```python
from build123d import *

# Parameters (mm, degrees)
SKETCH_223_R             = 11.5
SKETCH_223_R_2           = 8.5
EXTRUDE_6_DEPTH          = 11.5
SKETCH_7_R               = 11.5
EXTRUDE_7_DEPTH          = 15
CUT_EXTRUDE_1_REACH      = 36.373
CUT_EXTRUDE_1_END_RADIUS = 11.5
SKETCH_4_W               = 5
SKETCH_4_H               = 10
SKETCH_1_W               = 35
SKETCH_1_H               = 26.5
SKETCH_1_W_2             = 27
SKETCH_1_H_2             = 63
SKETCH_1_R               = 2.5
EXTRUDE_8_DEPTH          = 1.5
SKETCH_1_5_W             = 27
SKETCH_1_5_H             = 63
SKETCH_1_5_W_2           = 35
SKETCH_1_5_H_2           = 26.5
EXTRUDE_9_DEPTH          = 25
SKETCH_1_6_R             = 2.5
SKETCH_1_6_R_2           = 1.25
EXTRUDE_10_DEPTH         = 8
EXTRUDE_11_DEPTH         = 15
SKETCH_1_9_R             = 2
SKETCH_1_9_R_2           = 1.25
EXTRUDE_22_DEPTH         = 15
CUT_EXTRUDE_2_REACH      = 81.456
SKETCH_5_W               = 28
SKETCH_5_H               = 13
CUT_EXTRUDE_3_REACH      = 81.687
SKETCH_6_W               = 25
SKETCH_6_H               = 13
CUT_EXTRUDE_4_REACH      = 98.628


with BuildPart() as part:
    # Sketch 223 → Extrude 6 (new body)
    with BuildSketch(Plane(origin=(0, 0, 0), x_dir=(1, 0, 0), z_dir=(0, 1, 0))):
        with Locations(Location((14, 14, 0), (0, 0, 270))):
            Circle(SKETCH_223_R)
        with Locations(Location((14, 14, 0), (0, 0, 270))):
            Circle(SKETCH_223_R_2, mode=Mode.SUBTRACT)
    extrude(amount=EXTRUDE_6_DEPTH)

    # Sketch 7 → Extrude 7 (add)
    with BuildSketch(Plane(origin=(0, 0, 0), x_dir=(1, 0, 0), z_dir=(0, 1, 0))):
        with Locations(Location((14, 14, 0), (0, 0, 270))):
            Circle(SKETCH_7_R)
        with BuildLine():
            ThreePointArc((21.892872757, 19.724077187), (23.274103983, 17.008902675), (23.75, 14))
            ThreePointArc((23.75, 14), (21.390430568, 7.640437435), (15.453787483, 4.358993727))
            ThreePointArc((15.453787483, 4.358993727), (13.954467258, 3.002614207), (12.466429945, 4.371362356))
            ThreePointArc((12.466429945, 4.371362356), (4.976803671, 10.306163512), (6.1547961, 19.789237926))
            ThreePointArc((6.1547961, 19.789237926), (6.255870441, 21.80852258), (8.275922813, 21.892872757))
            ThreePointArc((8.275922813, 21.892872757), (14.040367815, 23.749916432), (19.789237926, 21.8452039))
            ThreePointArc((19.789237926, 21.8452039), (21.80852258, 21.744129559), (21.892872757, 19.724077187))
        make_face(mode=Mode.SUBTRACT)
    extrude(amount=EXTRUDE_7_DEPTH)

    # Cut-Extrude 1: up to this cylinder (the profile starts inside it)
    cut_extrude_1_end = Plane(origin=(14, 5, -14), z_dir=(0, -1, 0)) * Cylinder(CUT_EXTRUDE_1_END_RADIUS, 96.746, mode=Mode.PRIVATE)
    # Sketch 4 → Cut-Extrude 1 (cut, up to the surface)
    with BuildSketch(Plane.XY.offset(-20), mode=Mode.PRIVATE) as cut_extrude_1_sk1:
        with Locations((14.03258037, 5)):
            Rectangle(SKETCH_4_W, SKETCH_4_H)
    cut_extrude_1_tool1 = extrude(cut_extrude_1_sk1.sketch, amount=-CUT_EXTRUDE_1_REACH, mode=Mode.PRIVATE) & cut_extrude_1_end
    add(cut_extrude_1_tool1.solids().sort_by_distance((14.03258, 5, -20))[0], mode=Mode.SUBTRACT)

    # Sketch 1 → Extrude 8 (add)
    # profile 1 of 3: a face of its own
    with BuildSketch(Plane(origin=(0, 0, 0), x_dir=(1, 0, 0), z_dir=(0, 1, 0))):
        with Locations((19, 51.25)):
            Rectangle(SKETCH_1_W, SKETCH_1_H)
    # profile 2 of 3: a face of its own
    with BuildSketch(Plane(origin=(0, 0, 0), x_dir=(1, 0, 0), z_dir=(0, 1, 0))):
        with BuildLine():
            ThreePointArc((3.5, 37), (4.914213562, 33.585786438), (1.5, 35))
            Line((1.5, 35), (1.5, 3.5))
            ThreePointArc((1.5, 3.5), (4.914213562, 4.914213562), (3.5, 1.5))
            Line((3.5, 1.5), (34.5, 1.5))
            ThreePointArc((34.5, 1.5), (33.085786438, 4.914213562), (36.5, 3.5))
            Line((36.5, 3.5), (36.5, 35))
            ThreePointArc((36.5, 35), (33.085786438, 33.585786438), (34.5, 37))
            Line((34.5, 37), (3.5, 37))
        make_face()
    # profile 3 of 3: a face of its own
    with BuildSketch(Plane(origin=(0, 0, 0), x_dir=(1, 0, 0), z_dir=(0, 1, 0))):
        with Locations((51, 33)):
            Rectangle(SKETCH_1_W_2, SKETCH_1_H_2)
        with Locations(Location((40.9, 15.6, 0), (0, 0, 270))):
            Circle(SKETCH_1_R, mode=Mode.SUBTRACT)
        with Locations(Location((61.1, 15.6, 0), (0, 0, 270))):
            Circle(SKETCH_1_R, mode=Mode.SUBTRACT)
        with Locations(Location((40.9, 61.1, 0), (0, 0, 270))):
            Circle(SKETCH_1_R, mode=Mode.SUBTRACT)
        with Locations(Location((61.1, 61.1, 0), (0, 0, 270))):
            Circle(SKETCH_1_R, mode=Mode.SUBTRACT)
    extrude(amount=EXTRUDE_8_DEPTH)


with BuildPart() as extrude_8_piece_1:
    # of the separate pieces the step leaves, piece 1, a body of its own (extrude_8_pieces)
    add(part.part.solids().sort_by_distance((14, 15, -2.5))[0])



with BuildPart() as extrude_8_piece_2:
    # of the separate pieces the step leaves, piece 2, a body of its own (extrude_8_pieces)
    add(part.part.solids().sort_by_distance((37.5, 0, -1.5))[0])



with BuildPart() as extrude_8_piece_3:
    # of the separate pieces the step leaves, piece 3, a body of its own (extrude_8_pieces)
    add(part.part.solids().sort_by_distance((1.5, 0, -64.5))[0])


with BuildPart() as extrude_8_piece_2_1:
    add(extrude_8_piece_2.part)

    add(extrude_8_piece_3.part)  # Extrude 9 merges Extrude 8 piece 3
    # Sketch 1_5 → Extrude 9 (add)
    with BuildSketch(Plane(origin=(0, 0, 0), x_dir=(1, 0, 0), z_dir=(0, 1, 0))):
        Polygon((0, 37), (36.5, 37), (36.5, 0), (66, 0), (66, 66), (0, 66), align=None)
        with Locations((51, 33)):
            Rectangle(SKETCH_1_5_W, SKETCH_1_5_H, mode=Mode.SUBTRACT)
        with Locations((19, 51.25)):
            Rectangle(SKETCH_1_5_W_2, SKETCH_1_5_H_2, mode=Mode.SUBTRACT)
    extrude(amount=EXTRUDE_9_DEPTH)

    # Sketch 1_6 → Extrude 10 (add)
    # profile 1 of 4: a face of its own
    with BuildSketch(Plane(origin=(0, 0, 0), x_dir=(1, 0, 0), z_dir=(0, 1, 0))):
        with Locations(Location((61.1, 61.1, 0), (0, 0, 270))):
            Circle(SKETCH_1_6_R)
        with Locations(Location((61.1, 61.1, 0), (0, 0, 270))):
            Circle(SKETCH_1_6_R_2, mode=Mode.SUBTRACT)
    # profile 2 of 4: a face of its own
    with BuildSketch(Plane(origin=(0, 0, 0), x_dir=(1, 0, 0), z_dir=(0, 1, 0))):
        with Locations(Location((40.9, 61.1, 0), (0, 0, 270))):
            Circle(SKETCH_1_6_R)
        with Locations(Location((40.9, 61.1, 0), (0, 0, 270))):
            Circle(SKETCH_1_6_R_2, mode=Mode.SUBTRACT)
    # profile 3 of 4: a face of its own
    with BuildSketch(Plane(origin=(0, 0, 0), x_dir=(1, 0, 0), z_dir=(0, 1, 0))):
        with Locations(Location((40.9, 15.6, 0), (0, 0, 270))):
            Circle(SKETCH_1_6_R)
        with Locations(Location((40.9, 15.6, 0), (0, 0, 270))):
            Circle(SKETCH_1_6_R_2, mode=Mode.SUBTRACT)
    # profile 4 of 4: a face of its own
    with BuildSketch(Plane(origin=(0, 0, 0), x_dir=(1, 0, 0), z_dir=(0, 1, 0))):
        with Locations(Location((61.1, 15.6, 0), (0, 0, 270))):
            Circle(SKETCH_1_6_R)
        with Locations(Location((61.1, 15.6, 0), (0, 0, 270))):
            Circle(SKETCH_1_6_R_2, mode=Mode.SUBTRACT)
    extrude(amount=EXTRUDE_10_DEPTH)


with BuildPart() as extrude_8_piece_1_1:
    add(extrude_8_piece_1.part)

    add(extrude_8_piece_2_1.part)  # Extrude 11 merges Extrude 8 piece 2
    # Sketch 1_7 → Extrude 11 (add)
    with BuildSketch(Plane(origin=(0, 0, 0), x_dir=(1, 0, 0), z_dir=(0, 1, 0))):
        Polygon((1.5, 35), (1.5, 37), (0, 37), (0, 0), (36.5, 0), (36.5, 1.5), (34.5, 1.5), (3.5, 1.5), (1.5, 1.5), (1.5, 3.5), align=None)
    extrude(amount=EXTRUDE_11_DEPTH)

    # Sketch 1_9 → Extrude 22 (add)
    # profile 1 of 8: a face of its own
    with BuildSketch(Plane(origin=(0, 0, 0), x_dir=(1, 0, 0), z_dir=(0, 1, 0))):
        with Locations((3.5, 3.5)):
            Circle(SKETCH_1_9_R)
        with Locations(Location((3.5, 3.5, 0), (0, 0, 270))):
            Circle(SKETCH_1_9_R_2, mode=Mode.SUBTRACT)
    # profile 2 of 8: a face of its own
    with BuildSketch(Plane(origin=(0, 0, 0), x_dir=(1, 0, 0), z_dir=(0, 1, 0))):
        with BuildLine():
            ThreePointArc((3.5, 1.5), (2.085786438, 2.085786438), (1.5, 3.5))
            Line((1.5, 3.5), (1.5, 1.5))
            Line((1.5, 1.5), (3.5, 1.5))
        make_face()
    # profile 3 of 8: a face of its own
    with BuildSketch(Plane(origin=(0, 0, 0), x_dir=(1, 0, 0), z_dir=(0, 1, 0))):
        with Locations((34.5, 3.5)):
            Circle(SKETCH_1_9_R)
        with Locations(Location((34.5, 3.5, 0), (0, 0, 270))):
            Circle(SKETCH_1_9_R_2, mode=Mode.SUBTRACT)
    # profile 4 of 8: a face of its own
    with BuildSketch(Plane(origin=(0, 0, 0), x_dir=(1, 0, 0), z_dir=(0, 1, 0))):
        with BuildLine():
            ThreePointArc((36.5, 3.5), (35.914213562, 2.085786438), (34.5, 1.5))
            Line((34.5, 1.5), (36.5, 1.5))
            Line((36.5, 1.5), (36.5, 3.5))
        make_face()
    # profile 5 of 8: a face of its own
    with BuildSketch(Plane(origin=(0, 0, 0), x_dir=(1, 0, 0), z_dir=(0, 1, 0))):
        with Locations((34.5, 35)):
            Circle(SKETCH_1_9_R)
        with Locations(Location((34.5, 35, 0), (0, 0, 270))):
            Circle(SKETCH_1_9_R_2, mode=Mode.SUBTRACT)
    # profile 6 of 8: a face of its own
    with BuildSketch(Plane(origin=(0, 0, 0), x_dir=(1, 0, 0), z_dir=(0, 1, 0))):
        with BuildLine():
            Line((36.5, 37), (34.5, 37))
            ThreePointArc((34.5, 37), (35.914213562, 36.414213562), (36.5, 35))
            Line((36.5, 35), (36.5, 37))
        make_face()
    # profile 7 of 8: a face of its own
    with BuildSketch(Plane(origin=(0, 0, 0), x_dir=(1, 0, 0), z_dir=(0, 1, 0))):
        with Locations((3.5, 35)):
            Circle(SKETCH_1_9_R)
        with Locations(Location((3.5, 35, 0), (0, 0, 270))):
            Circle(SKETCH_1_9_R_2, mode=Mode.SUBTRACT)
    # profile 8 of 8: a face of its own
    with BuildSketch(Plane(origin=(0, 0, 0), x_dir=(1, 0, 0), z_dir=(0, 1, 0))):
        with BuildLine():
            Line((3.5, 37), (1.5, 37))
            Line((1.5, 37), (1.5, 35))
            ThreePointArc((1.5, 35), (2.085786438, 36.414213562), (3.5, 37))
        make_face()
    extrude(amount=EXTRUDE_22_DEPTH)

    # Sketch 5 → Cut-Extrude 2 (cut, up to next)
    with BuildSketch(Plane.ZY.offset(-36.5), mode=Mode.PRIVATE) as cut_extrude_2_sk1:
        with Locations((-18.5, 8)):
            Rectangle(SKETCH_5_W, SKETCH_5_H)
    cut_extrude_2_tool1 = extrude(cut_extrude_2_sk1.sketch, amount=-CUT_EXTRUDE_2_REACH, mode=Mode.PRIVATE) & extrude_8_piece_1_1.part
    add(cut_extrude_2_tool1.solids().sort_by_distance((36.5, 8, -18.5))[0], mode=Mode.SUBTRACT)

    # Sketch 6 → Cut-Extrude 3 (cut, up to next)
    with BuildSketch(Plane.XY.offset(-37), mode=Mode.PRIVATE) as cut_extrude_3_sk1:
        with Locations((20, 8)):
            Rectangle(SKETCH_6_W, SKETCH_6_H)
    cut_extrude_3_tool1 = extrude(cut_extrude_3_sk1.sketch, amount=-CUT_EXTRUDE_3_REACH, mode=Mode.PRIVATE) & extrude_8_piece_1_1.part
    add(cut_extrude_3_tool1.solids().sort_by_distance((20, 8, -37))[0], mode=Mode.SUBTRACT)

    # Sketch 7 2 → Cut-Extrude 4 (cut, up to next)
    with BuildSketch(Plane.ZY, mode=Mode.PRIVATE) as cut_extrude_4_sk1:
        with BuildLine():
            Line((-57.5, 10.5), (-45.5, 10.5))
            ThreePointArc((-45.5, 10.5), (-43, 8), (-45.5, 5.5))
            Line((-45.5, 5.5), (-57.5, 5.5))
            ThreePointArc((-57.5, 5.5), (-60, 8), (-57.5, 10.5))
        make_face()
    cut_extrude_4_tool1 = extrude(cut_extrude_4_sk1.sketch, amount=-CUT_EXTRUDE_4_REACH, mode=Mode.PRIVATE) & extrude_8_piece_1_1.part
    add(cut_extrude_4_tool1.solids().sort_by_distance((0, 8, -51.5))[0], mode=Mode.SUBTRACT)


solid = extrude_8_piece_1_1.part
```
Read the model definition and answer for the solid it produces. Units are mm, in the model's axes. A direction names the side the tool comes from. Coordinates: 2 decimals unless noted, no trailing zeros. Loops run counter-clockwise (first coordinate to the right, second up) from the corner with the lowest first, then second, coordinate; pieces in that order, holes last.
(1) A tool of negligible diameter and unlimited length cuts with its end or side. For faces 3 (the face through (11.533, 6, -24)), 4 (the face through (17.45, 8.16, -3.03)), 5 (the face through (1, 10.5, -52)), from which of +Z, -Z, +X, -X, +Y, -Y can it reach the whole face along a straight path? Write none if from no direction.
Solution:
face 3: none
face 4: +Y
face 5: -X
(2) The part is cut by section D-D (x = 50). Determine the outline of the cut face in (y, z).
Solution:
outline: (0, -66) - (25, -66) - (25, -64.5) - (1.5, -64.5) - (1.5, -1.5) - (25, -1.5) - (25, 0) - (0, 0) - close
(3) Flat-ended cylindrical pins translate along their axes: pin 1 Ø4 at (x, z) = (62, -15.5) entering from +Y; pin 2 Ø5 at (y, z) = (5, -58.5) entering from -X; pin 3 Ø1.2 at (x, z) = (35, -36) entering from +Y; pin 4 Ø10 at (x, z) = (22.5, -47.5) entering from +Y. Find the tip coordinate at first contact, or state that the pin passes through.
Solution:
pin 1: stops at y = 8
pin 2: stops at x = 0
pin 3: stops at y = 15
pin 4: stops at y = 1.5
(4) The part is cut by section A-A (y = 16). Determine the outline of the cut face in (x, z), and give its area (3 significant figures).
Solution:
outline: (0, -66) - (66, -66) - (66, 0) - (36.5, 0) - (36.5, -37) - (0, -37) - close; hole (1.5, -64.5) - (36.5, -64.5) - (36.5, -38) - (1.5, -38) - close; hole (37.5, -64.5) - (64.5, -64.5) - (64.5, -1.5) - (37.5, -1.5) - close
area: 377 mm2
(5) The mould has two halves that part along Z. Classify faces 1 (the face through (33, 0, -33)), 2 (the face through (42.14, 3.94, -61.26)): released by +Z, released by -Z, zero draft, split by the parting line, or undercut.
Solution:
face 1: zero draft
face 2: undercut
(6) Consider line 1 along X through (y, z) = (17, -61); line 2 along Z through (x, y) = (14, 9); line 3 along X through (y, z) = (16.75, -36). Determine where each line is inside the solid, lowest interval first.
Solution:
line 1: x = 0 to 1.5, 36.5 to 37.5, 64.5 to 66
line 2: z = -66 to -64.5, -5.5 to -2.5, -1.5 to 0
line 3: x = 36.5 to 37.5, 64.5 to 66
(7) The part is cut by section B-B (z = -48). Determine the outline of the cut face in (x, y).
Solution:
outline: (0, 0) - (66, 0) - (66, 25) - (64.5, 25) - (64.5, 1.5) - (37.5, 1.5) - (37.5, 25) - (36.5, 25) - (36.5, 1.5) - (1.5, 1.5) - (1.5, 5.5) - (0, 5.5) - close; (0, 10.5) - (1.5, 10.5) - (1.5, 25) - (0, 25) - close
(8) The part is cut by section C-C (x = 14). Determine the outline of the cut face in (y, z), and give its area (3 significant figures).
Solution:
outline: (0, -66) - (25, -66) - (25, -64.5) - (1.5, -64.5) - (1.5, -5.5) - (11.5, -5.5) - (11.5, -3) - (15, -3) - (15, -2.5) - (1.5, -2.5) - (1.5, -1.5) - (15, -1.5) - (15, 0) - (0, 0) - close; (10, -25.5) - (15, -25.5) - (15, -23.75) - (11.5, -23.75) - (11.5, -22.5) - (10, -22.5) - close; (14.5, -38) - (25, -38) - (25, -37) - (14.5, -37) - close
area: 207 mm2
